```python
from build123d import *

# Parameters (mm, degrees)
F0_W     = 25.4
F0_H     = 25.4
F0_W_2   = 19.05
F0_H_2   = 19.05
F1_DEPTH = 304.8
F2_W     = 25.4
F2_H     = 25.4
F3_DEPTH = 127
F4_R     = 3.2512
F5_DEPTH = 25.401


with BuildPart() as f1:
    # F0 (on Front) → F1 (new body, symmetric)
    with BuildSketch(Plane.XZ):
        Rectangle(F0_W, F0_H)
        Rectangle(F0_W_2, F0_H_2, mode=Mode.SUBTRACT)
    extrude(amount=F1_DEPTH, both=True)

    # F2 (on face) → F3 (join)
    with BuildSketch(Plane.YZ.offset(12.7)):
        Rectangle(F2_W, F2_H)
    extrude(amount=F3_DEPTH)

    # F4 (on face) → F5 (cut, through all)
    with BuildSketch(Plane.XY.offset(12.7)):
        Circle(F4_R)
        with Locations((123.8504, 0)):
            Circle(F4_R)
        with Locations((0, -111.1504)):
            Circle(F4_R)
    extrude(amount=-F5_DEPTH, mode=Mode.SUBTRACT)


solid = f1.part
```
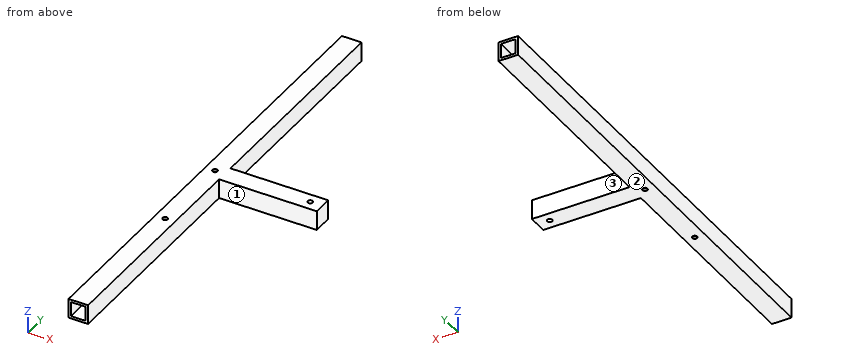
Geometry check sheet. Reference: the model listing, model coordinates, mm. Face numbers are marked on the shaded views. A direction names the side the tool comes from. Give positions to 0.01 mm unless a question says otherwise; leave off trailing zeros. Write each loop counter-clockwise with the first axis right and the second up, starting at its lowest first coordinate (ties: lowest second). Pieces come first, ordered by that corner, then holes.
1) Access from +Z, -Z, +X, -X, +Y, -Y to the whole of each face (thin tool, end or side, straight path). Record for the marked faces 1, 2 and 3.
2) Section check B-B, the plane y = 161. Record the boundary of the cut face in (x, z) (3 decimals), and give its area (3 significant figures).
3) Gauge pin test, flat ends, axial feed: pin 1 (5 mm diameter, centred on x = 107.5, z = 7, fed in from -Y); pin 2 (7.5 mm diameter, centred on y = -106, z = 4, fed in from +X); pin 3 (1.5 mm diameter, centred on x = 119, z = 6, fed in from +Y); pin 4 (7.5 mm diameter, centred on x = 0, y = -111.15, fed in from +Z). Record the tip position at first contact, or that the pin passes through.
4) Section check A-A, the plane z = -1.75. Record the boundary of the cut face in (x, y) (3 decimals).
5) Section check C-C, the plane x = 87.5. Record the boundary of the cut face in (y, z), and give its area (3 significant figures).
6) Material ranges on L1, parallel to Y at x = 0, z = -10.75; L2, parallel to X at y = 122, z = 2 (3 decimals), recorded low to high.
Computed:
1. face 1: +Z, -Z, +X, -Y
1. face 2: -Z, +X, -X, +Y, -Y
1. face 3: +Z, -Z, +X, +Y
2. outline: (-12.7, -12.7) - (12.7, -12.7) - (12.7, 12.7) - (-12.7, 12.7) - close; hole (-9.525, -9.525) - (9.525, -9.525) - (9.525, 9.525) - (-9.525, 9.525) - close
2. area: 282 mm2
3. pin 1: stops at y = -12.7
3. pin 2: stops at x = 12.7
3. pin 3: stops at y = 12.7
3. pin 4: stops at z = 12.7
4. outline: (-12.7, -304.8) - (-9.525, -304.8) - (-9.525, 304.8) - (-12.7, 304.8) - close; (9.525, -304.8) - (12.7, -304.8) - (12.7, -12.7) - (139.7, -12.7) - (139.7, 12.7) - (12.7, 12.7) - (12.7, 304.8) - (9.525, 304.8) - close; hole circle Ø6.502 at (123.85, 0)
5. outline: (-12.7, -12.7) - (12.7, -12.7) - (12.7, 12.7) - (-12.7, 12.7) - close
5. area: 645 mm2
6. L1: y = -304.8 to -114.4, -107.9 to -3.25, 3.25 to 304.8
6. L2: x = -12.7 to -9.525, 9.525 to 12.7
